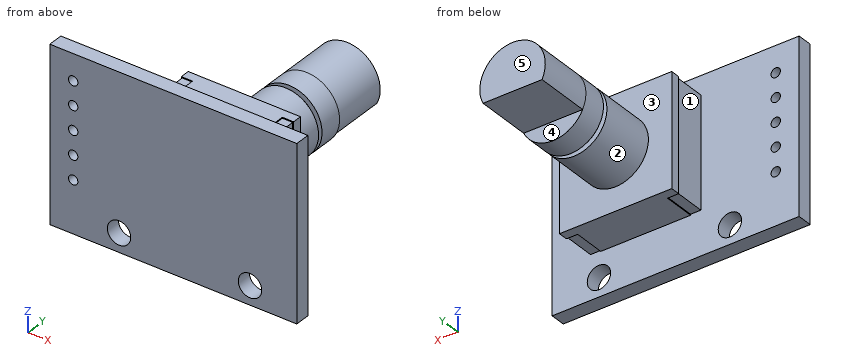
from build123d import *

# Parameters (mm, degrees)
SKETCH1_W           = 26.4
SKETCH1_H           = 18.5
SKETCH1_R           = 1.25
SKETCH1_R_2         = 0.5
BOSS_EXTRUDE1_DEPTH = 1.6
SKETCH2_W           = 12
SKETCH2_H           = 12
BOSS_EXTRUDE2_DEPTH = 4.35
CUT_EXTRUDE1_DEPTH  = 3.35
SKETCH4_R           = 3.5
BOSS_EXTRUDE3_DEPTH = 6
SKETCH5_R           = 2.967094381
BOSS_EXTRUDE4_DEPTH = 0.5
SKETCH6_R           = 3.5
BOSS_EXTRUDE5_DEPTH = 2.54
BOSS_EXTRUDE6_DEPTH = 5.88


with BuildPart() as part:
    # Sketch1 → Boss-Extrude1 (new body)
    with BuildSketch(Plane(origin=(0, 0, 0), x_dir=(1, 0, 0), z_dir=(0, 1, 0))):
        Rectangle(SKETCH1_W, SKETCH1_H)
        with Locations((-5.8, 7.25)):
            Circle(SKETCH1_R, mode=Mode.SUBTRACT)
        with Locations((8.2, 7.25)):
            Circle(SKETCH1_R, mode=Mode.SUBTRACT)
        with Locations((-10.7, -6.45)):
            Circle(SKETCH1_R_2, mode=Mode.SUBTRACT)
        with Locations((-10.7, -3.91)):
            Circle(SKETCH1_R_2, mode=Mode.SUBTRACT)
        with Locations((-10.7, -1.37)):
            Circle(SKETCH1_R_2, mode=Mode.SUBTRACT)
        with Locations((-10.7, 1.17)):
            Circle(SKETCH1_R_2, mode=Mode.SUBTRACT)
        with Locations((-10.7, 3.71)):
            Circle(SKETCH1_R_2, mode=Mode.SUBTRACT)
    extrude(amount=BOSS_EXTRUDE1_DEPTH)

    # Sketch2 → Boss-Extrude2 (add)
    with BuildSketch(Plane(origin=(0, 1.6, 0), x_dir=(1, 0, 0), z_dir=(0, 1, 0))):
        with Locations((3.2, -1.35)):
            Rectangle(SKETCH2_W, SKETCH2_H)
    extrude(amount=BOSS_EXTRUDE2_DEPTH)

    # Sketch3 → Cut-Extrude1 (cut)
    with BuildSketch(Plane(origin=(0, 1.6, 0), x_dir=(1, 0, 0), z_dir=(0, 1, 0))):
        Polygon((-1.6, 4.65), (-2.8, 4.65), (-2.8, -7.35), (-1.6, -7.35), (-1.6, -7.25), (-2.7, -7.25), (-2.7, 4.55), (-1.6, 4.55), align=None)
        Polygon((8, -7.35), (8, -7.25), (9.1, -7.25), (9.1, 4.55), (8, 4.55), (8, 4.65), (9.2, 4.65), (9.2, -7.35), align=None)
    extrude(amount=CUT_EXTRUDE1_DEPTH, mode=Mode.SUBTRACT)

    # Sketch4 → Boss-Extrude3 (add)
    with BuildSketch(Plane(origin=(0, 5.95, 0), x_dir=(1, 0, 0), z_dir=(0, 1, 0))):
        with Locations((3.2, -1.35)):
            Circle(SKETCH4_R)
    extrude(amount=BOSS_EXTRUDE3_DEPTH)

    # Sketch5 → Boss-Extrude4 (add)
    with BuildSketch(Plane(origin=(0, 11.95, 0), x_dir=(1, 0, 0), z_dir=(0, 1, 0))):
        with Locations((3.2, -1.35)):
            Circle(SKETCH5_R)
    extrude(amount=BOSS_EXTRUDE4_DEPTH)

    # Sketch6 → Boss-Extrude5 (add)
    with BuildSketch(Plane(origin=(0, 12.45, 0), x_dir=(1, 0, 0), z_dir=(0, 1, 0))):
        with Locations((3.2, -1.35)):
            Circle(SKETCH6_R)
    extrude(amount=BOSS_EXTRUDE5_DEPTH)

    # Sketch7 → Boss-Extrude6 (add)
    with BuildSketch(Plane(origin=(0, 14.99, 0), x_dir=(1, 0, 0), z_dir=(0, 1, 0))):
        with BuildLine():
            Line((0.047286883, 0.17), (6.352713117, 0.17))
            ThreePointArc((6.352713117, 0.17), (3.2, -4.85), (0.047286883, 0.17))
        make_face()
    extrude(amount=BOSS_EXTRUDE6_DEPTH)


solid = part.part
Can you work these out from the model? Positions are in its coordinate system, mm. Face numbers are marked on the shaded views. A direction names the side the tool comes from. Give positions to 0.01 mm unless a question says otherwise; leave off trailing zeros. Write each loop counter-clockwise with the first axis right and the second up, starting at its lowest first coordinate (ties: lowest second). Pieces come first, ordered by that corner, then holes. Notation, with made-up numbers: (77, 69.25) -> (117, 69.25) arc R23 cw to (117, 85.25) -> close; hole circle Ø3 at (28, -14.5). An arc over 180 degrees is marked (long way). Answer as a JSON object with one key per item and string values. Group by question number.
Item 1: I'm going to push flat-ended pins straight in: P1, Ø1.3, axis at x = 2.5, y = 3.5, coming from the +Z side; P2, Ø3.5, axis at y = 4, z = 0.5, coming from the +X side; P3, Ø4, axis at x = 2, y = 17.5, coming from the +Z side; P4, Ø1.5, axis at y = 9.5, z = 6, coming from the -X side. Where does each tip first touch, or does it pass through?
Item 2: Suppose I cut it at B-B (z = -3.71). Please give me the cut outline in (x, y), plus the area to 3 significant figures.
Item 3: For the marked faces 4 and 5, which set-ups out of +Z, -Z, +X, -X, +Y, -Y let a thin tool reach every point of the face, with its end or its side?
Item 4: We'd pull the mould along Y, two halves only. Please class the marked faces 1, 2 and 3: +Y half, -Y half, draft (parallel to the pull), parting line (faces both ways), or undercut.
Item 5: Suppose I cut it at A-A (x = -5.8). Please give me the cut outline in (y, z), plus the area to 3 significant figures.
Item 6: Suppose I cut it at C-C (x = -2.25). Please give me the cut outline in (y, z).
Item 7: Suppose I cut it at D-D (y = 3.75). Please give me the cut outline in (x, z), plus the area to 3 significant figures.
Item 8: Please list where these lines run through material, in increasing order: line 1 (X direction, y = 0.9, z = -7.25); line 2 (Z direction, x = -10.7, y = 1.2); line 3 (X direction, y = 1.1, z = -3.71). Write a range as [from, to].
Findings:
{
 "1": {"P1": "stops at z = 7.35", "P2": "stops at x = 9.2", "P3": "stops at z = 4.85", "P4": "passes through"},
 "2": {"outline": "(-13.2, 0) -> (-11.2, 0) -> (-11.2, 1.6) -> (-13.2, 1.6) -> close; (-10.2, 0) -> (13.2, 0) -> (13.2, 1.6) -> (9.1, 1.6) -> (9.1, 4.95) -> (9.2, 4.95) -> (9.2, 5.95) -> (-2.8, 5.95) -> (-2.8, 4.95) -> (-2.7, 4.95) -> (-2.7, 1.6) -> (-10.2, 1.6) -> close", "area": "92.2 mm²"},
 "3": {"face 4": "-Z, +X, -X, +Y", "face 5": "+Z, -Z, +X, -X, +Y"},
 "4": {"face 1": "undercut", "face 2": "draft", "face 3": "+Y half"},
 "5": {"outline": "(0, -9.25) -> (1.6, -9.25) -> (1.6, -8.5) -> (0, -8.5) -> close; (0, -6) -> (1.6, -6) -> (1.6, 9.25) -> (0, 9.25) -> close", "area": "25.6 mm²"},
 "6": {"outline": "(0, -9.25) -> (1.6, -9.25) -> (1.6, -4.55) -> (4.95, -4.55) -> (4.95, -4.65) -> (5.95, -4.65) -> (5.95, 7.35) -> (4.95, 7.35) -> (4.95, 7.25) -> (1.6, 7.25) -> (1.6, 9.25) -> (0, 9.25) -> close"},
 "7": {"outline": "(-2.7, -4.55) -> (-1.6, -4.55) -> (-1.6, -4.65) -> (8, -4.65) -> (8, -4.55) -> (9.1, -4.55) -> (9.1, 7.25) -> (8, 7.25) -> (8, 7.35) -> (-1.6, 7.35) -> (-1.6, 7.25) -> (-2.7, 7.25) -> close", "area": "141 mm²"},
 "8": {"line 1": "x = [-13.2, -7.05], [-4.55, 6.95], [9.45, 13.2]", "line 2": "z = [-9.25, -4.21], [-3.21, -1.67], [-0.67, 0.87], [1.87, 3.41], [4.41, 5.95], [6.95, 9.25]", "line 3": "x = [-13.2, -11.2], [-10.2, 13.2]"}
}
